Could you check a few things on this model? Use its own coordinates, in mm. Round coordinates to 2 decimals unless told otherwise and drop trailing zeros. Loops run counter-clockwise (first coordinate to the right, second up) from the corner with the lowest first, then second, coordinate; pieces in that order, holes last. Notation, with made-up numbers: (89.25, 3) -> (95.25, 3) arc R12 ccw to (95.25, 15) -> close; hole circle Ø4 at (6, 54). An arc over 180 degrees is marked (long way). Use CSV: the item, a comma, the result in double quotes. Start each with the question number.
```python
from build123d import *

# Parameters (mm, degrees)
BOSS_EXTRUDE1_DEPTH = 171
SKETCH2_R           = 1.25
CUT_EXTRUDE1_DEPTH  = 10
SKETCH4_R           = 1.25
CUT_EXTRUDE2_DEPTH  = 10
LPATTERN1_COUNT     = 7
LPATTERN1_PITCH     = 25.5
SKETCH5_W           = 6
SKETCH5_H           = 6
CUT_EXTRUDE3_DEPTH  = 10
LPATTERN2_COUNT     = 19
LPATTERN2_PITCH     = 9


with BuildPart() as part:
    # Sketch1 → Boss-Extrude1 (new body)
    with BuildSketch(Plane.XY):
        Polygon((-7.560747901, -2.297203345), (8.76644945, -1.788652997), (9.457807768, -2.612581756), (12.482904169, -0.866041535), (13.082904169, -1.905272019), (9.185789852, -4.155272019), (8.221608437, -3.006205355), (-6.986662858, -3.479904024), (-8.845450789, -5.695121219), (-12.742565106, -3.445121219), (-12.142565106, -2.405890734), (-9.117468705, -4.152430955), align=None)
    extrude(amount=BOSS_EXTRUDE1_DEPTH)

    # Sketch2 → Cut-Extrude1 (cut)
    with BuildSketch(Plane(origin=(3.495733027, -6.054787213, 0), x_dir=(0.8660254037844403, 0.49999999999999734, 0), z_dir=(-0.49999999999999734, 0.8660254037844403, 0))):
        with Locations(Location((8.377491356, -162, 0), (0, 0, 180))):
            Circle(SKETCH2_R)
    cut_extrude1 = extrude(amount=-CUT_EXTRUDE1_DEPTH, mode=Mode.SUBTRACT)

    # Sketch4 → Cut-Extrude2 (cut)
    with BuildSketch(Plane(origin=(-4.077422524, -7.062302975, 0), x_dir=(0.8660254037844392, -0.49999999999999917, 0), z_dir=(0.49999999999999917, 0.8660254037844392, 0))):
        with Locations(Location((-7.312824482, -162, 0), (0, 0, 180))):
            Circle(SKETCH4_R)
    cut_extrude2 = extrude(amount=-CUT_EXTRUDE2_DEPTH, mode=Mode.SUBTRACT)

    # LPattern1: Cut-Extrude1, Cut-Extrude2 ×7
    with Locations(*[(0, 0, -i * LPATTERN1_PITCH) for i in range(1, LPATTERN1_COUNT)]):
        add(cut_extrude1, mode=Mode.SUBTRACT)
        add(cut_extrude2, mode=Mode.SUBTRACT)

    # Sketch5 → Cut-Extrude3 (cut)
    with BuildSketch(Plane(origin=(0.064154599, -2.059707176, 0), x_dir=(0.9995152712604761, 0.031132338766899612, 0), z_dir=(-0.031132338766899612, 0.9995152712604761, 0))):
        with Locations((2.406515149, -166.5)):
            Rectangle(SKETCH5_W, SKETCH5_H)
    cut_extrude3 = extrude(amount=-CUT_EXTRUDE3_DEPTH, mode=Mode.SUBTRACT)

    # LPattern2: Cut-Extrude3 ×19
    with Locations(*[(0, 0, -i * LPATTERN2_PITCH) for i in range(1, LPATTERN2_COUNT)]):
        add(cut_extrude3, mode=Mode.SUBTRACT)


solid = part.part
```
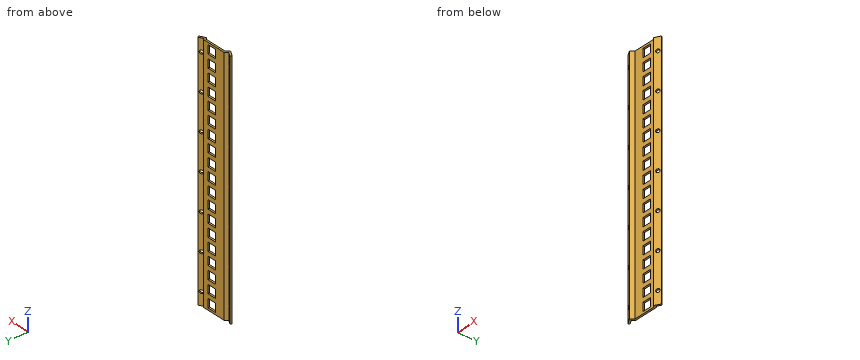
1. Will this pin go through, and if not, where does the flat tip stop? pin 1 (2 mm diameter, centred on x = 4.5, z = 135, fed in from -Y).
2. If I drill on L1, parallel to X at y = -2.75, z = 123.5; L2, parallel to Y at x = -0.75, z = 123.5; L3, parallel to X at y = -3.55, z = 76, over which ranges is the centre line in solid material (lowest first)?
3. Suppose I cut it at B-B (x = -4). List the corners of the cut face in (y, z) for me, then the cut area to 3 significant figures.
4. Suppose I cut it at A-A (z = 13.5). List the corners of the cut face in (x, y) for me, then the cut area to 3 significant figures.
Geometry check:
1,pin 1,"stops at y = -3.15"
2,L1,"x = -12.34 to -11.55, -7.94 to -0.51, 5.49 to 11.62"
2,L2,"y = -3.29 to -2.09"
2,L3,"x = -12.56 to -10.16, -8.61 to -7.05, 8.68 to 10.23"
3,outline,"(-3.39, 0) -> (-2.19, 0) -> (-2.19, 171) -> (-3.39, 171) -> close"
3,area,"205 mm²"
4,outline,"(-12.74, -3.45) -> (-8.85, -5.7) -> (-6.99, -3.48) -> (-0.49, -3.28) -> (-0.53, -2.08) -> (-7.56, -2.3) -> (-9.12, -4.15) -> (-12.14, -2.41) -> close; (5.47, -1.89) -> (5.51, -3.09) -> (8.22, -3.01) -> (9.19, -4.16) -> (13.08, -1.91) -> (12.48, -0.87) -> (9.46, -2.61) -> (8.77, -1.79) -> close"
4,area,"26.1 mm²"
